Here's how the part is built. I have some questions about the finished solid (model axes, mm). A direction names the side the tool comes from. Coordinates: 2 decimals unless noted, no trailing zeros. Write each loop counter-clockwise with the first axis right and the second up, starting at its lowest first coordinate (ties: lowest second). Pieces come first, ordered by that corner, then holes.
(1) Thinking about a two-plate mould opening in Z: for faces 4 (the cylindrical face through (35.786, -0.099, 19.748)), 5 (the conical face through (36.7, -1.62, 19.27)), 6 (the flat face through (14, -17.2, -19.1)), 7 (the cylindrical face through (8.169, -20.633, -15.821)), which applies, released by +Z, released by -Z, zero draft, split by the parting line, or undercut?
(2) Which directions (+Z, -Z, +X, -X, +Y, -Y) give clear straight access to the entire face, cutting with the end or side of a thin tool? Please do faces 1 (the flat face through (2.5, 1, 27)), 2 (the cylindrical face through (1.27, 34.23, 0.29)), 3 (the cylindrical face through (36.014, 11.923, 3.755)).
(3) Imagine slicing it at B-B, the plane y = 0. State how many separate pieces and enclosed holes the cut face has, plus the area to 3 significant figures.
(4) Imagine slicing it at C-C, the plane x = 4. List the corners of the cut face in (y, z) for me.
(5) Imagine slicing it at A-A, the plane z = 32. List the corners of the cut face in (x, y) for me, plus the area to 3 significant figures.
(6) Imagine slicing it at D-D, the plane y = 28. List the corners of the cut face in (x, z) for me, plus the area to 3 significant figures.
(7) Please list where these lines run through material, in increasing order: probe 1 along X at (y, z) = (19.5, -28.5); probe 2 along Z at (x, y) = (35.55, 17.5); probe 3 along Y at (x, z) = (2, 34).
(8) For pin 1 Ø1.5 at (x, y) = (11, -4.5) entering from -Z; pin 2 Ø2 at (x, y) = (17.5, 0.5) entering from +Z; pin 3 Ø6 at (x, y) = (30.5, 6) entering from +Z; pin 4 Ø3.5 at (y, z) = (17.5, 0) entering from +X, each with a flat end and sliding along its axis, tell me the tip position at first contact or that it passes through.
```python
from build123d import *

# Parameters (mm, degrees)
CSK_FOR_M4_FLAT_HEAD_MACHINE_SCREW1_AT_2_COUNT = 2
CSK_FOR_M4_FLAT_HEAD_MACHINE_SCREW1_AT_2_PITCH = 24.748737342
CSK_FOR_M4_FLAT_HEAD_MACHINE_SCREW1_AT_3_COUNT = 2
CSK_FOR_M4_FLAT_HEAD_MACHINE_SCREW1_AT_3_PITCH = 35
CSK_FOR_M4_FLAT_HEAD_MACHINE_SCREW1_AT_4_COUNT = 2
CSK_FOR_M4_FLAT_HEAD_MACHINE_SCREW1_AT_4_PITCH = 24.748737342
M4_CLEARANCE_HOLE1_D                           = 4.5
M4_CLEARANCE_HOLE1_DEPTH                       = 2.5
FILLET1_R                                      = 0.5


with BuildPart() as part:
    # Sketch2 → Revolve1 (revolve)
    with BuildSketch(Plane.XY):
        Polygon((0, 21), (35, 21), (35, 12.5), (37, 12.5), (37, 8.5), (39, 8.5), (39, 25), (14, 25), (14, 26), (2.5, 26), (2.5, 39), (0, 39), (0, 26), align=None)
    revolve(axis=Axis((-64.103352454, 0, 0), (1, 0, 0)))

    # Sketch8 → CSK for M4 Flat Head Machine Screw1 (revolve, cut)
    with BuildSketch(Plane(origin=(39, 17.5, 0), x_dir=(0, 0, -1), z_dir=(0, 1, 0))):
        Polygon((0, 0), (0, 4), (2.25, 4), (2.25, 2.45), (4.7, 0), align=None)
    csk_for_m4_flat_head_machine_screw1 = revolve(axis=Axis((45.35, 17.5, 0), (-1, 0, 0)), mode=Mode.SUBTRACT)

    # CSK for M4 Flat Head Machine Screw1 at 2: CSK for M4 Flat Head Machine Screw1 ×2
    with Locations(*[Vector(0, -0.707106781, -0.707106781) * (i * CSK_FOR_M4_FLAT_HEAD_MACHINE_SCREW1_AT_2_PITCH) for i in range(1, CSK_FOR_M4_FLAT_HEAD_MACHINE_SCREW1_AT_2_COUNT)]):
        add(csk_for_m4_flat_head_machine_screw1, mode=Mode.SUBTRACT)

    # CSK for M4 Flat Head Machine Screw1 at 3: CSK for M4 Flat Head Machine Screw1 ×2
    with Locations(*[(0, -i * CSK_FOR_M4_FLAT_HEAD_MACHINE_SCREW1_AT_3_PITCH, 0) for i in range(1, CSK_FOR_M4_FLAT_HEAD_MACHINE_SCREW1_AT_3_COUNT)]):
        add(csk_for_m4_flat_head_machine_screw1, mode=Mode.SUBTRACT)

    # CSK for M4 Flat Head Machine Screw1 at 4: CSK for M4 Flat Head Machine Screw1 ×2
    with Locations(*[Vector(0, -0.707106781, 0.707106781) * (i * CSK_FOR_M4_FLAT_HEAD_MACHINE_SCREW1_AT_4_PITCH) for i in range(1, CSK_FOR_M4_FLAT_HEAD_MACHINE_SCREW1_AT_4_COUNT)]):
        add(csk_for_m4_flat_head_machine_screw1, mode=Mode.SUBTRACT)

    # M4 Clearance Hole1
    with Locations(Plane.ZY):
        with Locations((0, 32), (0, -32), (32, 0), (-32, 0)):
            Hole(M4_CLEARANCE_HOLE1_D / 2, depth=M4_CLEARANCE_HOLE1_DEPTH)

    # Fillet1
    fillet1_edges = [part.edges().sort_by_distance(p)[0] for p in [
        (14, -25, 0),
    ]]
    fillet(fillet1_edges, radius=FILLET1_R)


solid = part.part
```
Recorded:
1. face 4: undercut
1. face 5: undercut
1. face 6: zero draft
1. face 7: split by the parting line
2. face 1: +X
2. face 2: +X, -X
2. face 3: -X
3. separate pieces: 6
3. enclosed holes: 0
3. area: 419 mm2
4. outline: circle Ø52 at (0, 0); hole circle Ø42 at (0, 0)
5. outline: (0, -22.29) - (2.5, -22.29) - (2.5, -2.25) - (0, -2.25) - close; (0, 2.25) - (2.5, 2.25) - (2.5, 22.29) - (0, 22.29) - close
5. area: 100 mm2
6. outline: (0, -27.15) - (2.5, -27.15) - (2.5, 27.15) - (0, 27.15) - close
6. area: 136 mm2
7. probe 1: x = 0 to 2.5
7. probe 2: z = -17.85 to -2.25, 2.25 to 17.85
7. probe 3: y = -19.1 to -1.03, 1.03 to 19.1
8. pin 1: stops at z = -25.73
8. pin 2: stops at z = 25
8. pin 3: stops at z = 24.82
8. pin 4: passes through
